from build123d import *

# Parameters (mm, degrees)
F0_R     = 4.7625
F1_DEPTH = 38.1
F3_DEPTH = 3.175


with BuildPart() as f1:
    # F0 (on Top) → F1 (new body)
    with BuildSketch(Plane.XY):
        Circle(F0_R)
    extrude(amount=F1_DEPTH)

    # F2 (on Front) → F3 (join, symmetric)
    with BuildSketch(Plane.XZ):
        with BuildLine():
            Line((2.669991, 24.872054), (13.890625, 29.575619))
            Line((13.890625, 29.575619), (13.890625, 32.907334))
            Line((13.890625, 32.907334), (2.669991, 37.610899))
            ThreePointArc((2.669991, 37.610899), (0, 38.147879), (-2.669991, 37.610899))
            Line((-2.669991, 37.610899), (-13.890625, 32.907334))
            Line((-13.890625, 32.907334), (-13.890625, 29.575619))
            Line((-13.890625, 29.575619), (-2.669991, 24.872054))
            ThreePointArc((-2.669991, 24.872054), (0, 24.335074), (2.669991, 24.872054))
        make_face()
    extrude(amount=F3_DEPTH, both=True)


solid = f1.part
Here's how the part is built. I have some questions about the finished solid (model axes, mm). A direction names the side the tool comes from. Coordinates: 2 decimals unless noted, no trailing zeros. Write each loop counter-clockwise with the first axis right and the second up, starting at its lowest first coordinate (ties: lowest second). Pieces come first, ordered by that corner, then holes.
1) Which directions (+Z, -Z, +X, -X, +Y, -Y) give clear straight access to the entire face, cutting with the end or side of a thin tool? Please do faces 1 (the face through (7, -3.175, 31)), 2 (the face through (7, 3.175, 31)), 3 (the face through (-8, -3.175, 31)).
Filled in:
face 1: +Z, -Z, +X, -Y
face 2: +Z, -Z, +X, +Y
face 3: +Z, -Z, -X, -Y
2) If we section it at B-B (y = -1.25): List the corners of the cut face in (x, z) for me, plus the area to 3 significant figures.
Filled in:
outline: (-13.89, 29.58) - (-4.6, 25.68) - (-4.6, 0) - (4.6, 0) - (4.6, 25.68) - (13.89, 29.58) - (13.89, 32.91) - (4.6, 36.8) - (4.6, 38.1) - (0.81, 38.1) arc R6.91 ccw to (-0.81, 38.1) - (-4.6, 38.1) - (-4.6, 36.8) - (-13.89, 32.91) - close
area: 485 mm2
3) If I drill on line 1 (Z direction, x = -4, y = 2.5); line 2 (X direction, y = 0.25, z = 13); line 3 (X direction, y = 3.75, z = 25.5), over which ranges is the centre line in solid material (lowest first)?
Filled in:
line 1: z = 0 to 38.1
line 2: x = -4.76 to 4.76
line 3: x = -2.94 to 2.94
4) I'm going to push flat-ended pins straight in: pin 1 (8.5 mm diameter, centred on x = 9.5, z = 32.5, fed in from -Y) (3 decimals); pin 2 (8.5 mm diameter, centred on x = -7.5, z = 31.5, fed in from -Y); pin 3 (3 mm diameter, centred on x = 3.5, y = -3.5, fed in from +Z). Where does each tip first touch, or does it pass through?
Filled in:
pin 1: stops at y = -3.175
pin 2: stops at y = -3.48
pin 3: stops at z = 38.1
5) If we section it at A-A (z = 34): List the corners of the cut face in (x, y) for me (1 decimal), plus the area to 3 significant figures.
Filled in:
outline: (-11.3, -3.2) - (-3.5, -3.2) arc R4.8 ccw to (3.5, -3.2) - (11.3, -3.2) - (11.3, 3.2) - (3.5, 3.2) arc R4.8 ccw to (-3.5, 3.2) - (-11.3, 3.2) - close
area: 159 mm2
6) If we section it at C-C (x = -12): List the corners of the cut face in (y, z) for me (3 decimals).
Filled in:
outline: (-3.175, 28.783) - (3.175, 28.783) - (3.175, 33.7) - (-3.175, 33.7) - close
7) If we section it at D-D (z = 13): List the corners of the cut face in (x, y) for me (1 decimal), plus the area to 3 significant figures.
Filled in:
outline: circle Ø9.5 at (0, 0)
area: 71.3 mm2
